```python
from build123d import *

# Parameters (mm, degrees)
SKETCH1_W           = 300
SKETCH1_H           = 100
BOSS_EXTRUDE1_DEPTH = 500
SHELL2_T            = 10
SKETCH2_W           = 300
SKETCH2_H           = 500
CUT_EXTRUDE1_DEPTH  = 10


with BuildPart() as part:
    # Sketch1 → Boss-Extrude1 (new body)
    with BuildSketch(Plane.XY):
        Rectangle(SKETCH1_W, SKETCH1_H)
    extrude(amount=BOSS_EXTRUDE1_DEPTH)

    # Shell2 (no face opened: a closed hollow body)
    add(offset(amount=-SHELL2_T, mode=Mode.PRIVATE), mode=Mode.SUBTRACT)

    # Sketch2 → Cut-Extrude1 (cut)
    with BuildSketch(Plane(origin=(0, 50, 0), x_dir=(1, 0, 0), z_dir=(0, 1, 0))):
        with Locations((0, -250)):
            Rectangle(SKETCH2_W, SKETCH2_H)
    extrude(amount=-CUT_EXTRUDE1_DEPTH, mode=Mode.SUBTRACT)


solid = part.part
```
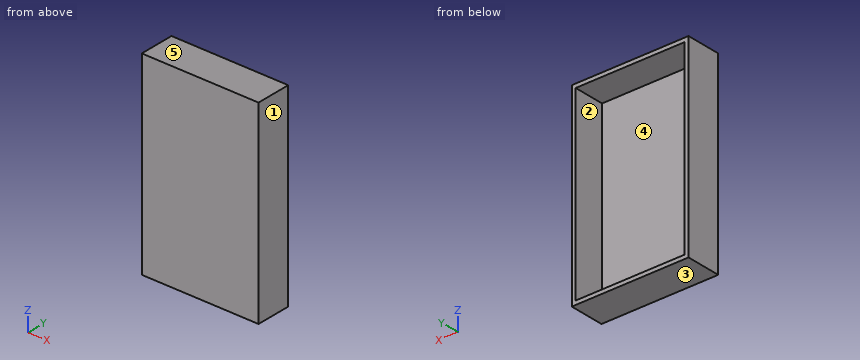
Geometry: final body of the model. Coordinates: model frame, mm. Face numbers are marked on the shaded views. A direction names the side the tool comes from. Round coordinates to 2 decimals unless told otherwise and drop trailing zeros. Loops run counter-clockwise (first coordinate to the right, second up) from the corner with the lowest first, then second, coordinate; pieces in that order, holes last. Notation, with made-up numbers: (11.25, -3.5) -> (51.25, -3.5) arc R30 ccw to (51.25, 20.5) -> close; hole circle Ø10 at (-36.5, -26.5). An arc over 180 degrees is marked (long way). Use one line per item in the form item = value.
Item 1: Cut plane B-B on y = 19. Output: boundary loops of the cut face in (x, z), then the cut area to 3 significant figures.
Evaluation:
outline = (-150, 0) -> (150, 0) -> (150, 500) -> (-150, 500) -> close; hole (-140, 10) -> (140, 10) -> (140, 490) -> (-140, 490) -> close
area = 15,600 mm2
Item 2: Contact query for a flat-ended pin moving along its axis: pin 1 Ø12 at (x, z) = (-51.5, 418) entering from +Y. Output: stop coordinate, or through.
Evaluation:
pin_1 = -40
Item 3: Cut plane A-A on z = 441.5. Output: boundary loops of the cut face in (x, y).
Evaluation:
outline = (-150, -50) -> (150, -50) -> (150, 40) -> (140, 40) -> (140, -40) -> (-140, -40) -> (-140, 40) -> (-150, 40) -> close
Item 4: Draft query along Z for the marked faces 1, 2 and 3. Return one class per face: released by +Z, released by -Z, zero draft, split by the parting line, or undercut.
Evaluation:
face_1 = zero draft
face_2 = undercut
face_3 = released by -Z
Item 5: Material intervals for probe 1 along X at (y, z) = (16.5, 390.5); probe 2 along Z at (x, y) = (110, 2); probe 3 along Y at (x, z) = (-20, 120.5), sorted ascending.
Evaluation:
probe_1 = -150 to -140, 140 to 150
probe_2 = 0 to 10, 490 to 500
probe_3 = -50 to -40
Item 6: Access query for the marked faces 4 and 5. Directions: +Z, -Z, +X, -X, +Y, -Y. A direction counts if a zero-diameter tool reaches every point of the face in a straight line with its end or side. Return the directions, or none.
Evaluation:
face_4 = +Y
face_5 = +Z, +X, -X, +Y, -Y
Item 7: Cut plane C-C on x = 78. Output: boundary loops of the cut face in (y, z), then the cut area to 3 significant figures.
Evaluation:
outline = (-50, 0) -> (40, 0) -> (40, 10) -> (-40, 10) -> (-40, 490) -> (40, 490) -> (40, 500) -> (-50, 500) -> close
area = 6,600 mm2
